```python
from build123d import *

# Parameters (mm, degrees)
F1_DEPTH = 152.4
F2_W     = 26.905142
F2_H     = 13.003318
F3_DEPTH = 25.4


with BuildPart() as f1:
    # F0 (on Front) → F1 (new body)
    with BuildSketch(Plane.XZ):
        with BuildLine():
            Line((7.62, 0), (0, 0))
            Line((0, 0), (0, -38.1))
            Line((0, -38.1), (38.1, -38.1))
            Line((38.1, -38.1), (38.1, 0))
            Line((38.1, 0), (30.48, 0))
            ThreePointArc((30.48, 0), (19.05, -7.108659), (7.62, 0))
        make_face()
    extrude(amount=-F1_DEPTH)

    # F2 (on face) → F3 (join)
    with BuildSketch(Plane(origin=(0, 0, 0), x_dir=(0, -1, 0), z_dir=(-1, 0, 0))):
        with Locations((-100.436237, -21.411889)):
            Rectangle(F2_W, F2_H)
    extrude(amount=F3_DEPTH)


solid = f1.part
```
Geometry check sheet. Reference: the model listing, model coordinates, mm. A direction names the side the tool comes from. Coordinates: 2 decimals unless noted, no trailing zeros. Order: outer loops, then holes, each group sorted by start corner. A loop starts at its lowest first (then second) coordinate and runs counter-clockwise, first axis right, second up.
Q1. Sectioned sample at A-A on y = 99. Record the cut outline in (x, z), and give its area (3 significant figures).
Reply:
outline: (-25.4, -27.91) - (0, -27.91) - (0, -38.1) - (38.1, -38.1) - (38.1, 0) - (30.48, 0) arc R12.74 cw to (7.62, 0) - (0, 0) - (0, -14.91) - (-25.4, -14.91) - close
area: 1,670 mm2
Q2. Sectioned sample at D-D on x = -17. Record the cut outline in (y, z), and give its area (3 significant figures).
Reply:
outline: (86.98, -27.91) - (113.89, -27.91) - (113.89, -14.91) - (86.98, -14.91) - close
area: 350 mm2
Q3. Sectioned sample at C-C on z = -19.5. Record the cut outline in (x, y).
Reply:
outline: (-25.4, 86.98) - (0, 86.98) - (0, 0) - (38.1, 0) - (38.1, 152.4) - (0, 152.4) - (0, 113.89) - (-25.4, 113.89) - close
Q4. Sectioned sample at B-B on z = -3.5. Record the cut outline in (x, y), and give its area (3 significant figures).
Reply:
outline: (0, 0) - (10.16, 0) - (10.16, 152.4) - (0, 152.4) - close; (27.94, 0) - (38.1, 0) - (38.1, 152.4) - (27.94, 152.4) - close
area: 3,100 mm2
Q5. Depth check by flat-ended pin: pin 1 Ø10 at (x, z) = (-9, -30.5) entering from +Y; pin 2 Ø14.5 at (x, z) = (-8.5, -24.5) entering from -Y; pin 3 Ø3 at (y, z) = (129.5, -8) entering from -X. Enter the tip coordinate at first touch or a pass-through.
Reply:
pin 1: stops at y = 113.89
pin 2: stops at y = 86.98
pin 3: stops at x = 0
Q6. Tool access check on faces 1 (the face through (-13, 86.984, -22)), 2 (the face through (-13, 113.889, -22)), 3 (the face through (-13, 101, -14.91)), 4 (the face through (-13, 101, -27.914)). Record the directions out of +Z, -Z, +X, -X, +Y, -Y that give a thin tool (end or side, any length) a straight path to the whole face; none if there is none.
Reply:
face 1: +Z, -Z, -X, -Y
face 2: +Z, -Z, -X, +Y
face 3: +Z, -X, +Y, -Y
face 4: -Z, -X, +Y, -Y
Q7. Thickness scan on probe 1 along X at (y, z) = (75, -27.5); probe 2 along Z at (x, y) = (-17, 103.5); probe 3 along Y at (x, z) = (-10, -20.5). Record the ranges inside material, lowest first.
Reply:
probe 1: x = 0 to 38.1
probe 2: z = -27.91 to -14.91
probe 3: y = 86.98 to 113.89
